Can you work these out from the model? Positions are in its coordinate system, mm. A direction names the side the tool comes from. Round coordinates to 2 decimals unless told otherwise and drop trailing zeros. Order: outer loops, then holes, each group sorted by start corner. A loop starts at its lowest first (then second) coordinate and runs counter-clockwise, first axis right, second up.
from build123d import *

# Parameters (mm, degrees)
SKETCH1_W                      = 41.4
SKETCH1_H                      = 15
SKETCH1_R                      = 1.1
BOSS_EXTRUDE1_DEPTH            = 5
SKETCH2_W                      = 41.4
SKETCH2_H                      = 4.8
BOSS_EXTRUDE2_DEPTH            = 5
CBORE_FOR_M2_SHCS1_D           = 2.2
CBORE_FOR_M2_SHCS1_CBORE_D     = 4.4
CBORE_FOR_M2_SHCS1_CBORE_DEPTH = 2
FILLET1_R                      = 5


with BuildPart() as part:
    # Sketch1 → Boss-Extrude1 (new body)
    with BuildSketch(Plane.XY):
        Rectangle(SKETCH1_W, SKETCH1_H)
        with Locations((-11.2, 5)):
            Circle(SKETCH1_R, mode=Mode.SUBTRACT)
        with Locations((12.8, 5)):
            Circle(SKETCH1_R, mode=Mode.SUBTRACT)
        with Locations(Location((12.8, -5, 0), (0, 0, 180))):
            Circle(SKETCH1_R, mode=Mode.SUBTRACT)
        with Locations(Location((-11.2, -5, 0), (0, 0, 180))):
            Circle(SKETCH1_R, mode=Mode.SUBTRACT)
    extrude(amount=BOSS_EXTRUDE1_DEPTH)

    # Sketch2 → Boss-Extrude2 (add)
    with BuildSketch(Plane.XY):
        Rectangle(SKETCH2_W, SKETCH2_H)
    extrude(amount=-BOSS_EXTRUDE2_DEPTH)

    # CBORE for M2 SHCS1 (through all)
    with Locations(Plane.XY.offset(5)):
        with Locations((-11.2, 5), (12.8, 5), (12.8, -5), (-11.2, -5)):
            CounterBoreHole(CBORE_FOR_M2_SHCS1_D / 2, CBORE_FOR_M2_SHCS1_CBORE_D / 2, CBORE_FOR_M2_SHCS1_CBORE_DEPTH)

    # Fillet1
    fillet1_edges = [part.edges().sort_by_distance(p)[0] for p in [
        (-20.7, 0, 5),
        (20.7, 0, 5),
    ]]
    fillet(fillet1_edges, radius=FILLET1_R - 0.0001)  # a hair under: the kernel refuses the full size


solid = part.part
(1) I want a section at B-B, the plane y = -5. Give the number of separate pieces and of enclosed holes in the cut face, plus the area to 3 significant figures.
(2) On a 3-axis mill with a long thin cutter (end or side, diameter ignored), from which of +Z, -Z, +X, -X, +Y, -Y can I reach the whole of each face in a straight line? I mean faces 4 (the face through (0, -2.4, -2)), 5 (the face through (0, 5, 0)), 6 (the face through (14.832, 4.157, 4.014)). Say none if no direction works.
(3) If we mould it in two halves opening along X, with no side actions, what happens to faces 1 (the face through (0, 0, -5)), 2 (the face through (19.27, 0.11, 3.5)), 3 (the face through (13.816, 4.579, 1.479))? For each: pulls with the +X half, pulls with the -X half, needs draft (parallel to the pull), parting line crosses it, or undercut.
(4) I want a section at D-D, the plane z = 1.75. List the corners of the cut face in (x, y) for me.
(5) I want a section at C-C, the plane x = -6. List the corners of the cut face in (y, z) for me, plus the area to 3 significant figures.
(6) I want a section at A-A, the plane x = 12.8. List the corners of the cut face in (y, z) for me.
(7) Please list where these lines run through material, in increasing order: probe 1 along Y at (x, z) = (-11.2, 4.6); probe 2 along Y at (x, z) = (-11.2, 1.15); probe 3 along X at (y, z) = (-5.5, 1).
(8) I'm going to push flat-ended pins straight in: pin 1 Ø2 at (x, y) = (6.5, 4) entering from -Z; pin 2 Ø3.5 at (x, y) = (-11.2, -5) entering from +Z; pin 3 Ø2.5 at (x, z) = (-6, -2.5) entering from -Y. Where does each tip first touch, or does it pass through?
Ans:
1. separate pieces: 3
1. enclosed holes: 0
1. area: 165 mm2
2. face 4: -Z, +X, -X, -Y
2. face 5: -Z, +X, -X, +Y
2. face 6: +Z
3. face 1: needs draft
3. face 2: pulls with the +X half
3. face 3: undercut
4. outline: (-20.38, -7.5) - (20.38, -7.5) - (20.38, 7.5) - (-20.38, 7.5) - close; hole circle Ø2.2 at (-11.2, -5); hole circle Ø2.2 at (-11.2, 5); hole circle Ø2.2 at (12.8, -5); hole circle Ø2.2 at (12.8, 5)
5. outline: (-7.5, 0) - (-2.4, 0) - (-2.4, -5) - (2.4, -5) - (2.4, 0) - (7.5, 0) - (7.5, 5) - (-7.5, 5) - close
5. area: 99.0 mm2
6. outline: (-7.5, 0) - (-6.1, 0) - (-6.1, 3) - (-7.2, 3) - (-7.2, 5) - (-7.5, 5) - close; (-3.9, 0) - (-2.4, 0) - (-2.4, -5) - (2.4, -5) - (2.4, 0) - (3.9, 0) - (3.9, 3) - (2.8, 3) - (2.8, 5) - (-2.8, 5) - (-2.8, 3) - (-3.9, 3) - close; (6.1, 0) - (7.5, 0) - (7.5, 5) - (7.2, 5) - (7.2, 3) - (6.1, 3) - close
7. probe 1: y = -7.5 to -7.2, -2.8 to 2.8, 7.2 to 7.5
7. probe 2: y = -7.5 to -6.1, -3.9 to 3.9, 6.1 to 7.5
7. probe 3: x = -20.6 to -12.18, -10.22 to 11.82, 13.78 to 20.6
8. pin 1: stops at z = 0
8. pin 2: stops at z = 3
8. pin 3: stops at y = -2.4
